The model under review builds one solid part; all positions refer to its coordinate system, in mm. Face numbers are marked on the shaded views. Give positions to 0.01 mm unless a question says otherwise; leave off trailing zeros. Order: outer loops, then holes, each group sorted by start corner. A loop starts at its lowest first (then second) coordinate and runs counter-clockwise, first axis right, second up. Notation, with made-up numbers: (-39.5, 50.25) -> (7.5, 50.25) arc R15 ccw to (7.5, 74.25) -> close; hole circle Ø10 at (62.25, 15). An arc over 180 degrees is marked (long way). Use one line per item in the form item = value.
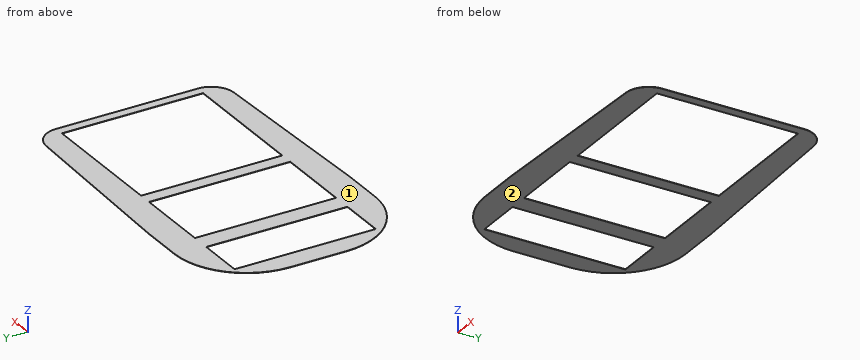
Autodesk Inventor part; units mm, degrees
ref_plane "YZ Plane" through (0, 0, 0) normal (1, 0, 0) x (0, 1, 0)
ref_plane "XZ Plane" through (0, 0, 0) normal (0, 1, 0) x (-1, 0, 0)
ref_plane "XY Plane" through (0, 0, 0) normal (0, 0, 1) x (1, 0, 0)
sketch "Sketch1" plane through (0, 0, 0) normal (0, 0, 1) x (1, 0, 0)
  arc A0 (216.4448, 899.4448) -> (-166.5552, 516.4448) centre (216.4448, 516.4448) ccw
  line L0 (-166.5552, 216.4448) -> (-166.5552, 516.4448)
  arc A1 (-166.5552, 216.4448) -> (216.4448, -166.5552) centre (216.4448, 216.4448) ccw
  line L1 (443.4448, -166.5552) -> (216.4448, -166.5552)
  line L2 (216.4448, 899.4448) -> (443.4448, 899.4448)
  line L3 (443.5712, 899.4425) -> (1403.908, 864.732)
  line L4 (1403.908, -131.8425) -> (443.5712, -166.5529)
  arc A2 (443.4448, -166.5552) -> (443.5712, -166.5529) centre (443.4448, -163.0552) ccw
  arc A3 (443.5712, 899.4425) -> (443.4448, 899.4448) centre (443.4448, 895.9448) ccw
  arc A4 (1521.5977, 742.7757) -> (1403.908, 864.732) centre (1399.4977, 742.7117) ccw
  line L5 (1521.5977, 742.7757) -> (1521.6067, 725.4805)
  line L6 (1521.6067, 7.4091) -> (1521.5977, -9.8861)
  arc A5 (1403.908, -131.8425) -> (1521.5977, -9.8861) centre (1399.4977, -9.8222) ccw
  line L7 (1521.6067, 725.4805) -> (1521.6067, 7.4091)
  point P0 (0, 0)
extrude "Plate1" add sketch "Sketch1" along normal blind 1.5
sketch "Sketch2" plane through (0, 0, 1.5) normal (0, 0, 1) x (1, 0, 0)
  line L0 (771.6067, -8.5552) -> (1471.6067, -8.5552)
  line L1 (1471.6067, -8.5552) -> (1471.6067, 741.4448)
  line L2 (1471.6067, 741.4448) -> (771.6067, 741.4448)
  line L3 (771.6067, 741.4448) -> (771.6067, -8.5552)
  arc A0 (443.5712, 899.4425) -> (443.4448, 899.4448) centre (443.4448, 895.9448) ccw
  line L4 (216.4448, 899.4448) -> (443.4448, 899.4448)
  arc A1 (216.4448, 899.4448) -> (-166.5552, 516.4448) centre (216.4448, 516.4448) ccw
  line L5 (-166.5552, 216.4448) -> (-166.5552, 516.4448)
  arc A2 (-166.5552, 216.4448) -> (216.4448, -166.5552) centre (216.4448, 216.4448) ccw
  line L6 (443.4448, -166.5552) -> (216.4448, -166.5552)
  arc A3 (443.4448, -166.5552) -> (443.5712, -166.5529) centre (443.4448, -163.0552) ccw
  line L7 (1403.908, -131.8425) -> (443.5712, -166.5529)
  arc A4 (1403.908, -131.8425) -> (1521.5977, -9.8861) centre (1399.4977, -9.8222) ccw
  line L8 (1521.6067, 7.4091) -> (1521.5977, -9.8861)
  line L9 (1521.6067, 725.4805) -> (1521.6067, 7.4091)
  line L10 (1521.5977, 742.7757) -> (1521.6067, 725.4805)
  arc A5 (1521.5977, 742.7757) -> (1403.908, 864.732) centre (1399.4977, 742.7117) ccw
  line L11 (443.5712, 899.4425) -> (1403.908, 864.732)
  line L12 (296.6067, -8.5552) -> (701.6067, -8.5552)
  line L13 (701.6067, -8.5552) -> (701.6067, 741.4448)
  line L14 (701.6067, 741.4448) -> (296.6067, 741.4448)
  line L15 (296.6067, 741.4448) -> (296.6067, -8.5552)
  line L16 (-53.3933, -8.5552) -> (196.6067, -8.5552)
  line L17 (196.6067, -8.5552) -> (196.6067, 741.4448)
  line L18 (196.6067, 741.4448) -> (-53.3933, 741.4448)
  line L19 (-53.3933, 741.4448) -> (-53.3933, -8.5552)
  point P0 (0, 0)
  point P1 (1471.6067, 366.4448)
  point P2 (1521.6067, 366.4448)
  point P3 (701.6067, 366.4448)
  point P4 (771.6067, 366.4448)
  point P5 (196.6067, 366.4448)
  point P6 (296.6067, 366.4448)
  dimension "d1" = 50
  dimension "d2" = 750
  dimension "d3" = 700
  dimension "d4" = 750
  dimension "d5" = 70
  dimension "d6" = 405
  dimension "d7" = 750
  dimension "d8" = 100
  dimension "d9" = 250
extrude "Extrusion1" cut sketch "Sketch2" against normal through all contours L3 L2 L1 L0 | L15 L14 L13 L12 | L19 L18 L17 L16
equation "\"d0\" = Thickness"
equation "\"BendRadius\" = Thickness"
equation "\"BendReliefWidth\" = Thickness"
equation "\"BendReliefDepth\" = 0.5 * Thickness"
equation "\"CornerReliefSize\" = 4 * Thickness"
equation "\"MinimumRemnant\" = 2 * Thickness"
equation "\"TransitionRadius\" = BendRadius"
equation "\"JacobiRadiusSize\" = BendRadius"
equation "\"GapSize\" = Thickness"
properties part number "CHAPA_6"
1. Add section C-C on z = 0.3. Give the boundary of the cut face in (x, y).
Values:
outline = (-166.56, 216.44) arc R383 ccw to (216.44, -166.56) -> (443.44, -166.56) arc R3.45 ccw to (443.57, -166.55) -> (1403.91, -131.84) arc R122.1 ccw to (1521.6, -9.89) -> (1521.61, 7.41) -> (1521.61, 725.48) -> (1521.6, 742.78) arc R122.1 ccw to (1403.91, 864.73) -> (443.57, 899.44) arc R3.55 ccw to (443.44, 899.44) -> (216.44, 899.44) arc R383 ccw to (-166.56, 516.44) -> close; hole (-53.39, -8.56) -> (196.61, -8.56) -> (196.61, 741.44) -> (-53.39, 741.44) -> close; hole (296.61, -8.56) -> (701.61, -8.56) -> (701.61, 741.44) -> (296.61, 741.44) -> close; hole (771.61, -8.56) -> (1471.61, -8.56) -> (1471.61, 741.44) -> (771.61, 741.44) -> close
2. Add section B-B on y = 405. Give the boundary of the cut face in (x, z), then the cut area to 3 significant figures.
Values:
outline = (-166.56, 0) -> (-53.39, 0) -> (-53.39, 1.5) -> (-166.56, 1.5) -> close; (196.61, 0) -> (296.61, 0) -> (296.61, 1.5) -> (196.61, 1.5) -> close; (701.61, 0) -> (771.61, 0) -> (771.61, 1.5) -> (701.61, 1.5) -> close; (1471.61, 0) -> (1521.61, 0) -> (1521.61, 1.5) -> (1471.61, 1.5) -> close
area = 500 mm^2
3. Add section A-A on x = 1324.5. Give the boundary of the cut face in (y, z).
Values:
outline = (-134.71, 0) -> (-8.56, 0) -> (-8.56, 1.5) -> (-134.71, 1.5) -> close; (741.44, 0) -> (867.6, 0) -> (867.6, 1.5) -> (741.44, 1.5) -> close
4. For L1, parallel to X at y = 216.5, z = 1.1; L2, parallel to X at y = 721, z = 1.25; L3, parallel to Y at x = 304, z = 1.2, list the stretches that pass through material, from the lowest coordinate up.
Values:
L1 = -166.56 to -53.39, 196.61 to 296.61, 701.61 to 771.61, 1471.61 to 1521.61
L2 = -107.35 to -53.39, 196.61 to 296.61, 701.61 to 771.61, 1471.61 to 1521.61
L3 = -166.56 to -8.56, 741.44 to 899.44
5. The part is to be moulded in two halves that separate along Z. For the marked faces 1 and 2, say which applies: +Z half, -Z half, draft (parallel to the pull), parting line (faces both ways), or undercut.
Values:
face_1 = +Z half
face_2 = -Z half
6. For pin 1 Ø0.8 at (x, z) = (1211.5, 1) entering from -Y, flat-tipped, find the tip position at first contact; note if it passes through.
Values:
pin_1 = -138.81
7. Add section D-D on y = 191.5. Give the boundary of the cut face in (x, z), then the cut area to 3 significant figures.
Values:
outline = (-165.74, 0) -> (-53.39, 0) -> (-53.39, 1.5) -> (-165.74, 1.5) -> close; (196.61, 0) -> (296.61, 0) -> (296.61, 1.5) -> (196.61, 1.5) -> close; (701.61, 0) -> (771.61, 0) -> (771.61, 1.5) -> (701.61, 1.5) -> close; (1471.61, 0) -> (1521.61, 0) -> (1521.61, 1.5) -> (1471.61, 1.5) -> close
area = 499 mm^2
